Source: CAD feature listing. Evaluate the final solid. Frame: model axes, mm. A direction names the side the tool comes from. Round coordinates to 2 decimals unless told otherwise and drop trailing zeros. Order: outer loops, then holes, each group sorted by start corner. A loop starts at its lowest first (then second) coordinate and runs counter-clockwise, first axis right, second up. Notation, with made-up numbers: (52.25, 10.5) -> (63.25, 10.5) arc R18 cw to (63.25, 17.5) -> close; hole circle Ø6 at (34, 32.5). An arc over 180 degrees is marked (long way). Answer as CSV lines item,"result". Start each with the question number.
(1) Line query: line 1 along Y through (x, z) = (0, 2.5); line 2 along Y through (x, z) = (0, 7.5); line 3 along Z through (x, y) = (-8.25, 5.25). Output: solid intervals per line, ascending. Write a range as from..to.
(2) Contact query for flat-ended pins moving along their axis: P1, Ø2, axis at x = 4, y = -0.5, coming from the +Z side; P2, Ø5.5, axis at x = 0, y = 8, coming from the +Z side; P3, Ø1.5, axis at y = -4, z = 7, coming from the +X side; P4, Ø5, axis at y = -3.5, z = 3, coming from the +X side. Output: stop coordinate, or through.
(3) Pull-direction query (Y, two-part tool) for faces 1 (the flat face through (2, -5, 5)), 2 (the cylindrical face through (2.4, -4.5, 0.7)), 3 (the cylindrical face through (9.669, 0.526, 3.226)); classes: +Y half, -Y half, draft (parallel to the pull), parting line (faces both ways), or undercut.
(4) Set-up query: faces 4 (the flat face through (2, -5, 1.5)), 5 (the cylindrical face through (2.4, -4.5, 9.9)), 6 (the cylindrical face through (0.534, 4.065, 7.395)). Return all of +Z, -Z, +X, -X, +Y, -Y with unobstructed straight access to the full face (end or side cutting, diameter ignored); none if empty.
(5) Section query A-A (x = 0). Output: boundary loops of the cut face in (y, z).
(6) Section query D-D (z = 4). Output: boundary loops of the cut face in (x, y).
(7) Section query C-C (x = -9). Output: boundary loops of the cut face in (y, z).
(8) Section query B-B (y = 7.25). Output: boundary loops of the cut face in (x, z), plus the area to 3 significant figures.
```python
from build123d import *

# Parameters (mm, degrees)
SKETCH1_R           = 5.1
BOSS_EXTRUDE1_DEPTH = 15
SKETCH2_R           = 11
SKETCH2_R_2         = 1.75
BOSS_EXTRUDE2_DEPTH = 3.5
SKETCH3_R           = 4.1
CUT_EXTRUDE1_DEPTH  = 22.610182785


with BuildPart() as part:
    # Sketch1 → Boss-Extrude1 (new body)
    with BuildSketch(Plane.XY):
        Circle(SKETCH1_R)
    extrude(amount=BOSS_EXTRUDE1_DEPTH)

    # Sketch2 → Boss-Extrude2 (add)
    with BuildSketch(Plane.XY.offset(1.5)):
        Circle(SKETCH2_R)
        with Locations((0, 8)):
            Circle(SKETCH2_R_2, mode=Mode.SUBTRACT)
        with Locations((8, 0)):
            Circle(SKETCH2_R_2, mode=Mode.SUBTRACT)
        with Locations((0, -8)):
            Circle(SKETCH2_R_2, mode=Mode.SUBTRACT)
        with Locations((-8, 0)):
            Circle(SKETCH2_R_2, mode=Mode.SUBTRACT)
    extrude(amount=BOSS_EXTRUDE2_DEPTH)

    # Sketch3 → Cut-Extrude1 (cut, through all)
    with BuildSketch(Plane(origin=(0, 0, 0), x_dir=(-1, 0, 0), z_dir=(0, 0, -1))):
        Circle(SKETCH3_R)
    extrude(amount=-CUT_EXTRUDE1_DEPTH, mode=Mode.SUBTRACT)


solid = part.part
```
Answer block:
1,line 1,"-11..-9.75, -6.25..-4.1, 4.1..6.25, 9.75..11"
1,line 2,"-5.1..-4.1, 4.1..5.1"
1,line 3,"1.5..5"
2,P1,"z = 15"
2,P2,"z = 5"
2,P3,"x = 3.93"
2,P4,"x = 10.95"
3,face 1,"draft"
3,face 2,"parting line"
3,face 3,"undercut"
4,face 4,"-Z"
4,face 5,"+Z"
4,face 6,"+Z, -Z"
5,outline,"(-11, 1.5) -> (-9.75, 1.5) -> (-9.75, 5) -> (-11, 5) -> close; (-6.25, 1.5) -> (-5.1, 1.5) -> (-5.1, 0) -> (-4.1, 0) -> (-4.1, 15) -> (-5.1, 15) -> (-5.1, 5) -> (-6.25, 5) -> close; (4.1, 0) -> (5.1, 0) -> (5.1, 1.5) -> (6.25, 1.5) -> (6.25, 5) -> (5.1, 5) -> (5.1, 15) -> (4.1, 15) -> close; (9.75, 1.5) -> (11, 1.5) -> (11, 5) -> (9.75, 5) -> close"
6,outline,"circle Ø22 at (0, 0); hole circle Ø3.5 at (-8, 0); hole circle Ø8.2 at (0, 0); hole circle Ø3.5 at (0, -8); hole circle Ø3.5 at (0, 8); hole circle Ø3.5 at (8, 0)"
7,outline,"(-6.32, 1.5) -> (-1.44, 1.5) -> (-1.44, 5) -> (-6.32, 5) -> close; (1.44, 1.5) -> (6.32, 1.5) -> (6.32, 5) -> (1.44, 5) -> close"
8,outline,"(-8.27, 1.5) -> (-1.58, 1.5) -> (-1.58, 5) -> (-8.27, 5) -> close; (1.58, 1.5) -> (8.27, 1.5) -> (8.27, 5) -> (1.58, 5) -> close"
8,area,"46.8 mm2"
